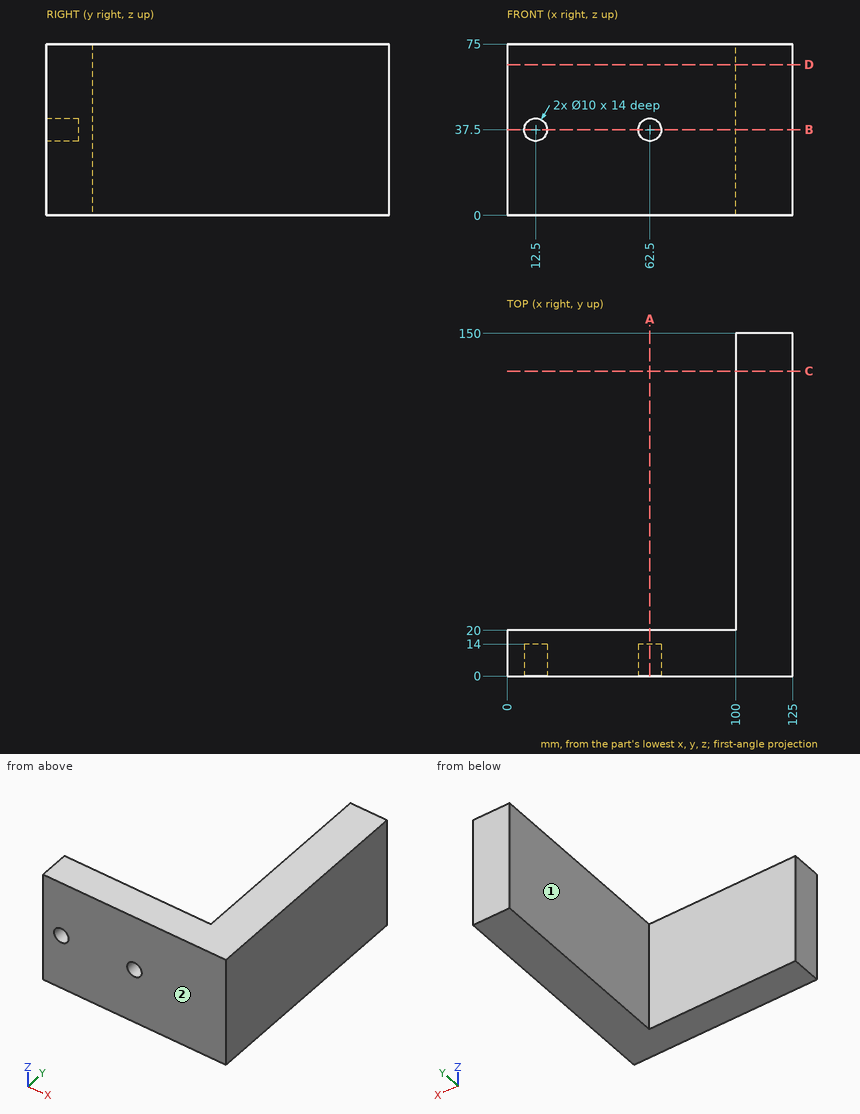
Study the drawing (mm; zero at the part's minimum x, y, z) and answer. A direction names the side the tool comes from. Give positions to 0.01 mm unless a question says otherwise; leave off trailing zeros. Write each loop counter-clockwise with the first axis right and the second up, starting at its lowest first coordinate (ties: lowest second). Pieces come first, ordered by that corner, then holes. Notation, with made-up numbers: (-15.5, 25) - (31.5, 25) arc R34 ccw to (31.5, 57) - close; hole circle Ø6 at (-6, 31.5). An arc over 180 degrees is marked (long way). Use CSV: the item, a comma, the result in double quotes. Start each with the question number.
(1) Given P1, Ø6, axis at x = 30, z = 18.5, coming from the +Y side; P2, Ø3, axis at x = 14, z = 35.5, coming from the -Y side; P3, Ø1, axis at y = 92, z = 8, coming from the -X side, each flat-ended and moving along its own axis, determine where each tip first touches the part or whether it passes through.
(2) Find section D-D (z = 66). Give the vertices of the cut face in (x, y).
(3) Consider line 1 along X through (y, z) = (8, 37); line 2 along X through (y, z) = (136, 58); line 3 along Y through (x, z) = (50, 54). Determine where each line is inside the solid, lowest interval first.
(4) Find section B-B (z = 37.5). Give the vertices of the cut face in (x, y).
(5) Find section C-C (y = 133.5). Give the vertices of the cut face in (x, z), plus the area to 4 significant figures.
(6) For the marked faces 1 and 2, determine the directions among +Z, -Z, +X, -X, +Y, -Y from which every point of the face is accessible in a straight line to the end or side of a thin tool.
(7) Find section A-A (x = 62.5). Give the vertices of the cut face in (y, z), plus the area to 3 significant figures.
Findings below:
1,P1,"y = 20"
1,P2,"y = 14"
1,P3,"x = 100"
2,outline,"(0, 0) - (125, 0) - (125, 150) - (100, 150) - (100, 20) - (0, 20) - close"
3,line 1,"0 to 7.53, 17.47 to 57.53, 67.47 to 125"
3,line 2,"100 to 125"
3,line 3,"0 to 20"
4,outline,"(0, 0) - (7.5, 0) - (7.5, 14) - (17.5, 14) - (17.5, 0) - (57.5, 0) - (57.5, 14) - (67.5, 14) - (67.5, 0) - (125, 0) - (125, 150) - (100, 150) - (100, 20) - (0, 20) - close"
5,outline,"(100, 0) - (125, 0) - (125, 75) - (100, 75) - close"
5,area,"1,875 mm2"
6,face 1,"+Z, -Z, -X, +Y"
6,face 2,"+Z, -Z, +X, -X, -Y"
7,outline,"(0, 0) - (20, 0) - (20, 75) - (0, 75) - (0, 42.5) - (14, 42.5) - (14, 32.5) - (0, 32.5) - close"
7,area,"1,360 mm2"
